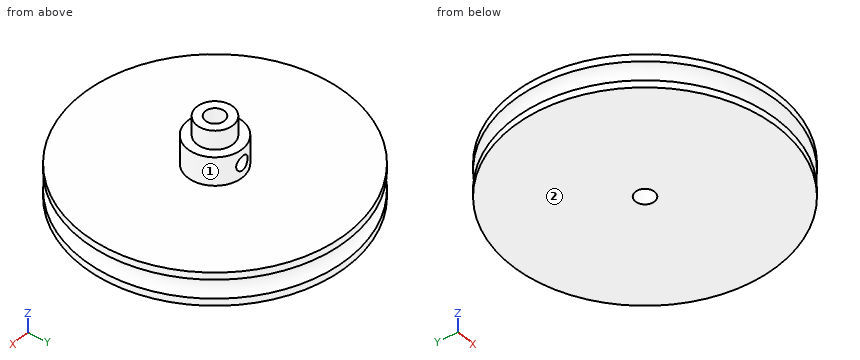
from build123d import *

# Parameters (mm, degrees)
ESQUISSE1_R             = 28
BOSS_EXTRU_1_DEPTH      = 7
ESQUISSE2_R             = 3.8
BOSS_EXTRU_2_DEPTH      = 10
ESQUISSE3_R             = 2
ENL_V_MAT_EXTRU_1_DEPTH = 18
ESQUISSE4_R             = 2
ESQUISSE5_R             = 5.75
ESQUISSE5_R_2           = 3.8
BOSS_EXTRU_3_DEPTH      = 6
ENL_V_MAT_EXTRU_2_REACH = 30
ESQUISSE6_R             = 1.5


with BuildPart() as part:
    # Esquisse1 → Boss.-Extru.1 (new body)
    with BuildSketch(Plane.XY):
        Circle(ESQUISSE1_R)
    extrude(amount=BOSS_EXTRU_1_DEPTH)

    # Esquisse2 → Boss.-Extru.2 (add)
    with BuildSketch(Plane.XY.offset(7)):
        Circle(ESQUISSE2_R)
    extrude(amount=BOSS_EXTRU_2_DEPTH)

    # Esquisse3 → Enlèv. mat.-Extru.1 (cut, through all)
    with BuildSketch(Plane.XY.offset(17)):
        Circle(ESQUISSE3_R)
    extrude(amount=-ENL_V_MAT_EXTRU_1_DEPTH, mode=Mode.SUBTRACT)

    # Esquisse4 → Enlèvement de matière-Révolution1 (revolve, cut)
    with BuildSketch(Plane(origin=(0, 0, 0), x_dir=(0, 0, -1), z_dir=(1, 0, 0))):
        with Locations((-3.5, 28)):
            Circle(ESQUISSE4_R)
    revolve(axis=Axis((0, 0, 0), (0, 0, 1)), mode=Mode.SUBTRACT)

    # Esquisse5 → Boss.-Extru.3 (add)
    with BuildSketch(Plane.XY.offset(7)):
        Circle(ESQUISSE5_R)
        Circle(ESQUISSE5_R_2, mode=Mode.SUBTRACT)
    extrude(amount=BOSS_EXTRU_3_DEPTH)

    # Esquisse6 → Enlèv. mat.-Extru.2 (cut, up to next)
    with BuildSketch(Plane(origin=(0, 0, 0), x_dir=(1, 0, 0), z_dir=(0, 1, 0)), mode=Mode.PRIVATE) as enl_v_mat_extru_2_sk1:
        with Locations((0, -10)):
            Circle(ESQUISSE6_R)
    enl_v_mat_extru_2_tool1 = extrude(enl_v_mat_extru_2_sk1.sketch, amount=ENL_V_MAT_EXTRU_2_REACH, mode=Mode.PRIVATE) & part.part
    add(enl_v_mat_extru_2_tool1.solids().sort_by_distance((0, 0, 10))[0], mode=Mode.SUBTRACT)


solid = part.part
Geometry check sheet. Reference: the model listing, model coordinates, mm. Face numbers are marked on the shaded views. A direction names the side the tool comes from. Coordinates: 2 decimals unless noted, no trailing zeros. Order: outer loops, then holes, each group sorted by start corner. A loop starts at its lowest first (then second) coordinate and runs counter-clockwise, first axis right, second up. Notation, with made-up numbers: (54, 36) - (58, 36) arc R20 cw to (58, 43) - close; hole circle Ø8 at (78.5, 82.25). An arc over 180 degrees is marked (long way). Answer in a Markdown table with one row per item. Add a question column.
1) Cross-section at A-A, the plane x = 0. Record the cut outline in (y, z), then the cut area to 3 significant figures.
2) Material ranges on line 1 along Z through (x, y) = (0, 2.35); line 2 along Y through (x, z) = (0, 12.25); line 3 along Z through (x, y) = (-12.5, 20), recorded low to high. Write a range as [from, to].
3) Cross-section at C-C, the plane z = 10. Record the cut outline in (x, y).
4) Cross-section at B-B, the plane z = 2.5. Record the cut outline in (x, y).
5) Set-up check for the marked faces 1 and 2: record each of +Z, -Z, +X, -X, +Y, -Y from which the full face is reachable in a straight line by a thin tool's end or side.
6) Gauge pin test, flat ends, axial feed: P1, Ø2, axis at x = 2.5, y = -19, coming from the +Z side; P2, Ø3, axis at x = -15.5, z = 3.5, coming from the -Y side; P3, Ø3.5, axis at x = 0, y = 0, coming from the -Z side; P4, Ø6, axis at x = -9.5, z = 4, coming from the +Y side. Record the tip position at first contact, or that the pin passes through.
Check result:
| question | item | result |
|---|---|---|
| 1 | outline | (-28, 0) - (-2, 0) - (-2, 17) - (-3.8, 17) - (-3.8, 13) - (-5.75, 13) - (-5.75, 7) - (-28, 7) - (-28, 5.5) arc R2 cw to (-28, 1.5) - close; (2, 0) - (28, 0) - (28, 1.5) arc R2 cw to (28, 5.5) - (28, 7) - (5.75, 7) - (5.75, 8.5) - (2, 8.5) - close; (2, 11.5) - (5.75, 11.5) - (5.75, 13) - (3.8, 13) - (3.8, 17) - (2, 17) - close |
| 1 | area | 400 mm² |
| 2 | line 1 | z = [0, 8.5], [11.5, 17] |
| 2 | line 2 | y = [-5.75, -2], [2, 5.75] |
| 2 | line 3 | z = [0, 7] |
| 3 | outline | (-1.5, 1.32) - (-1.5, 5.55) arc R5.75 ccw (long way) to (1.5, 5.55) - (1.5, 1.32) arc R2 cw (long way) to start |
| 4 | outline | circle Ø52.54 at (0, 0); hole circle Ø4 at (0, 0) |
| 5 | face 1 | +Z |
| 5 | face 2 | -Z, +X, -X, +Y, -Y |
| 6 | P1 | stops at z = 7 |
| 6 | P2 | stops at y = -22 |
| 6 | P3 | passes through |
| 6 | P4 | stops at y = 27.14 |
